Design review of the part built by this model. Coordinates are the model's own, in mm. A direction names the side the tool comes from. Round coordinates to 2 decimals unless told otherwise and drop trailing zeros. Loops run counter-clockwise (first coordinate to the right, second up) from the corner with the lowest first, then second, coordinate; pieces in that order, holes last. Notation, with made-up numbers: M 85,-19.75 L 122,-19.75 A9 cw 122,-3.75 Z; hole C -19,-33 d5. An arc over 180 degrees is marked long. One line per item, written item: value. Start each with the question number.
Item 1: For faces 4 (the flat face through (-1, 1, 1)), 5 (the flat face through (-3, 23, 29)), 6 (the flat face through (-24.571, 12, 29)), list the 3-axis set-ups (+Z, -Z, +X, -X, +Y, -Y) from which the entire face can be reached by the end or side of a thin tool; tool diameter is ignored.
Item 2: We need section B-B (z = -17.5). Write out the cut boundary in (x, y), then the cut area to 3 significant figures.
Item 3: For line 1 along X through (y, z) = (3.5, 23); line 2 along Z through (x, y) = (0.5, 18.5); line 3 along Y through (x, z) = (-22, -20.5), list the stretches that pass through material, from the lowest coordinate up.
Item 4: We need section C-C (y = 20.5). Write out the cut boundary in (x, z).
Item 5: Clearance check with a flat-ended pin moving along its axis: pin 1 (5 mm diameter, centred on x = 3.5, z = -11, fed in from +Y). State where the tip first meets the part, or that it passes through.
Item 6: We need section A-A (x = -22). Write out the cut boundary in (y, z), then the cut area to 3 significant figures.
Item 7: Mouldability with a two-part tool opening along Z and no side actions: class faces 1 (the flat face through (25.429, 5, 29)), 2 (the flat face through (0, 11, -27.944)), 3 (the flat face through (-1, 12, -26.444)) as released by +Z, released by -Z, zero draft, split by the parting line, or undercut.
Item 8: We need section D-D (x = 13.5). Write out the cut boundary in (y, z), then the cut area to 3 significant figures.
from build123d import *

# Parameters (mm, degrees)
BOSS_EXTRUDE2_DEPTH = 1
BOSS_EXTRUDE3_DEPTH = 23
SKETCH1_4_W         = 66
SKETCH1_4_H         = 1.5
BOSS_EXTRUDE4_DEPTH = 23
SKETCH5_W           = 10
SKETCH5_H           = 4
CUT_EXTRUDE3_DEPTH  = 10


with BuildPart() as part:
    # Sketch1 → Boss-Extrude2 (new body)
    with BuildSketch(Plane(origin=(0, 0, 0), x_dir=(1, 0, 0), z_dir=(0, 1, 0))):
        Polygon((-33.571389819, -30.056333369), (-33.571389819, -28.556333369), (32.428610181, -28.556333369), (32.428610181, -30.056333369), (33.928610181, -30.056333369), (33.928610181, 27.943666631), (-35.071389819, 27.943666631), (-35.071389819, -30.056333369), align=None)
    extrude(amount=BOSS_EXTRUDE2_DEPTH)

    # Sketch1<3> → Boss-Extrude3 (add)
    with BuildSketch(Plane(origin=(0, 0, 0), x_dir=(1, 0, 0), z_dir=(0, 1, 0))):
        Polygon((-33.571389819, -30.056333369), (-33.571389819, -28.556333369), (-33.571389819, 26.443666631), (32.428610181, 26.443666631), (32.428610181, -28.556333369), (32.428610181, -30.056333369), (33.928610181, -30.056333369), (33.928610181, 27.943666631), (-35.071389819, 27.943666631), (-35.071389819, -30.056333369), align=None)
    extrude(amount=BOSS_EXTRUDE3_DEPTH)

    # Sketch1<4> → Boss-Extrude4 (add)
    with BuildSketch(Plane(origin=(0, 0, 0), x_dir=(1, 0, 0), z_dir=(0, 1, 0))):
        with Locations((-0.571389819, -29.306333369)):
            Rectangle(SKETCH1_4_W, SKETCH1_4_H)
    extrude(amount=BOSS_EXTRUDE4_DEPTH)

    # Sketch5 → Cut-Extrude3 (cut)
    with BuildSketch(Plane.XY.offset(30.056333369)):
        with Locations((20.428610181, 5)):
            Rectangle(SKETCH5_W, SKETCH5_H)
        with Locations((-19.571389819, 12)):
            Rectangle(SKETCH5_W, SKETCH5_H)
    extrude(amount=-CUT_EXTRUDE3_DEPTH, mode=Mode.SUBTRACT)


solid = part.part
A:
1. face 4: +Y
1. face 5: +Z, -Z, +X, -X, +Y
1. face 6: +Z
2. outline: M -35.07,0 L 33.93,0 L 33.93,23 L 32.43,23 L 32.43,1 L -33.57,1 L -33.57,23 L -35.07,23 Z
2. area: 135 mm2
3. line 1: -35.07 to -33.57, 32.43 to 33.93
3. line 2: -27.94 to -26.44, 28.56 to 30.06
3. line 3: 0 to 1
4. outline: M -35.07,-27.94 L 33.93,-27.94 L 33.93,30.06 L -35.07,30.06 Z; hole M -33.57,-26.44 L 32.43,-26.44 L 32.43,28.56 L -33.57,28.56 Z
5. pin 1: y = 1
6. outline: M 0,-27.94 L 23,-27.94 L 23,-26.44 L 1,-26.44 L 1,28.56 L 10,28.56 L 10,30.06 L 0,30.06 Z; M 14,28.56 L 23,28.56 L 23,30.06 L 14,30.06 Z
6. area: 118 mm2
7. face 1: zero draft
7. face 2: released by -Z
7. face 3: undercut
8. outline: M 0,-27.94 L 23,-27.94 L 23,-26.44 L 1,-26.44 L 1,28.56 L 23,28.56 L 23,30.06 L 0,30.06 Z
8. area: 124 mm2
